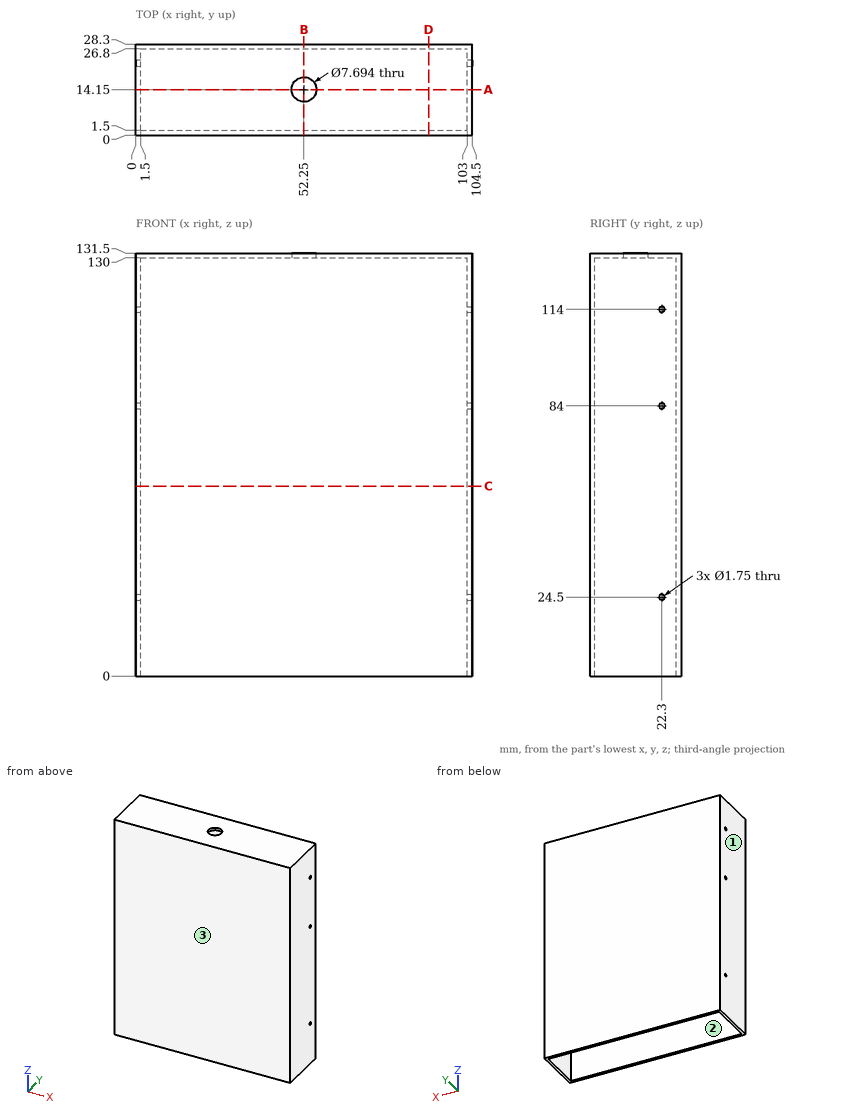
Verification items for this drawing (mm, ordinates from the low corner). Give positions to 0.01 mm unless a question says otherwise; leave off trailing zeros. Loops run counter-clockwise (first coordinate to the right, second up) from the corner with the lowest first, then second, coordinate; pieces in that order, holes last. Notation, with made-up numbers: M 39,-15.5 L 97,-15.5 A13 cw 97,-6.5 Z; hole C 15.25,-37.5 d5. An arc over 180 degrees is marked long. Return JSON: item names as keys, results as strings. Group by question number.
1. Go/stop test with flat-tipped pins: pin 1 (6 mm diameter, centred on y = 24, z = 45, fed in from -X); pin 2 (1.1 mm diameter, centred on y = 22.3, z = 24.5, fed in from -X); pin 3 (10 mm diameter, centred on x = 74, y = 20.5, fed in from -Z). Record where each tip stops, or that it passes through.
2. Cross-section at D-D on x = 91. Record the boundary of the cut face in (y, z).
3. Thickness scan on L1, parallel to Z at x = 103.85, y = 22.3 (3 decimals); L2, parallel to Y at x = 11.5, z = 34; L3, parallel to X at y = 26.75, z = 87. Record the ranges inside material, lowest first.
4. Mould release check, pull along Y, two halves, no side actions. Record for the marked faces 1, 2 and 3: released by +Y, released by -Y, zero draft, split by the parting line, or undercut.
5. Cross-section at C-C on z = 59. Record the boundary of the cut face in (x, y).
6. Cross-section at A-A on y = 14.15. Record the boundary of the cut face in (x, z), plus the area to 3 significant figures.
7. Cross-section at B-B on x = 52.25. Record the boundary of the cut face in (y, z).
Return value:
{
 "1": {"pin 1": "x = 0", "pin 2": "through", "pin 3": "z = 130"},
 "2": {"outline": "M 0,0 L 1.5,0 L 1.5,130 L 26.8,130 L 26.8,0 L 28.3,0 L 28.3,131.5 L 0,131.5 Z"},
 "3": {"L1": "0 to 23.625, 25.375 to 83.125, 84.875 to 113.125, 114.875 to 131.5", "L2": "0 to 1.5, 26.8 to 28.3", "L3": "0 to 1.5, 103 to 104.5"},
 "4": {"face 1": "zero draft", "face 2": "undercut", "face 3": "released by -Y"},
 "5": {"outline": "M 0,0 L 104.5,0 L 104.5,28.3 L 0,28.3 Z; hole M 1.5,1.5 L 103,1.5 L 103,26.8 L 1.5,26.8 Z"},
 "6": {"outline": "M 0,0 L 1.5,0 L 1.5,130 L 48.4,130 L 48.4,131.5 L 0,131.5 Z; M 56.1,130 L 103,130 L 103,0 L 104.5,0 L 104.5,131.5 L 56.1,131.5 Z", "area": "535 mm^2"},
 "7": {"outline": "M 0,0 L 1.5,0 L 1.5,130 L 10.3,130 L 10.3,131.5 L 0,131.5 Z; M 18,130 L 26.8,130 L 26.8,0 L 28.3,0 L 28.3,131.5 L 18,131.5 Z"}
}
